Design review of the part shown in the three views and the two pictorial views. Dimensions are in mm from the part's minimum x, y and z. A direction names the side the tool comes from. Round coordinates to 2 decimals unless told otherwise and drop trailing zeros. Loops run counter-clockwise (first coordinate to the right, second up) from the corner with the lowest first, then second, coordinate; pieces in that order, holes last. Notation, with made-up numbers: (-2.75, 55.25) - (11.25, 55.25) arc R20 ccw to (11.25, 84.25) - close; hole circle Ø8 at (82, -31). An arc over 180 degrees is marked (long way). Return JSON: item names as keys, results as strings. Group by question number.
(1) The part is to be moulded in two halves that separate along Z. For the marked faces 3, 4 and 5, say which applies: pulls with the +Z half, pulls with the -Z half, needs draft (parallel to the pull), parting line crosses it, or undercut.
(2) We need section B-B, the plane y = 11. Write out the cut boundary in (x, z), and give its area (3 significant figures).
(3) Clearance check with a flat-ended pin moving along its axis: pin 1 (5 mm diameter, centred on x = 59.5, y = 12, fed in from +Z). State where the tip first meets the part, or that it passes through.
(4) We need section A-A, the plane x = 86. Write out the cut boundary in (y, z).
(5) Wall thickness on L1, parallel to Z at x = 81, y = 4.5; L2, parallel to X at y = 21.25, z = 114.5; L3, parallel to Z at x = 22, y = 20.25: over which ranges is each line inside the solid? List them lowest first. Write a range as [from, to].
(6) We need section D-D, the plane z = 18. Write out the cut boundary in (x, y).
(7) We need section C-C, the plane x = 148. Write out the cut boundary in (y, z).
(8) For the marked faces 1 and 2, list the 3-axis set-ups (+Z, -Z, +X, -X, +Y, -Y) from which the entire face can be reached by the end or side of a thin tool; tool diameter is ignored.
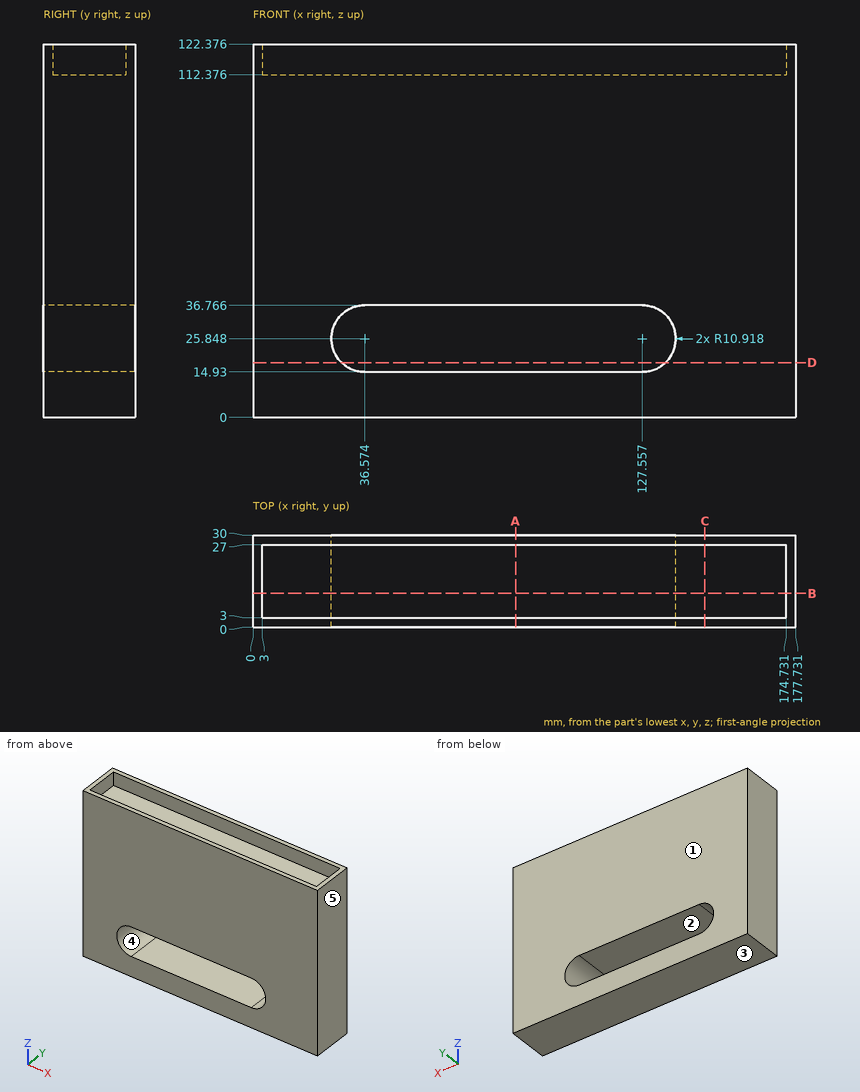
Solutions:
{
 "1": {"face 3": "pulls with the -Z half", "face 4": "undercut", "face 5": "needs draft"},
 "2": {"outline": "(0, 0) - (177.73, 0) - (177.73, 122.38) - (174.73, 122.38) - (174.73, 112.38) - (3, 112.38) - (3, 122.38) - (0, 122.38) - close; hole (36.57, 14.93) - (127.56, 14.93) arc R10.92 ccw to (127.56, 36.77) - (36.57, 36.77) arc R10.92 ccw to start", "area": "17,700 mm^2"},
 "3": {"pin 1": "z = 112.38"},
 "4": {"outline": "(0, 0) - (30, 0) - (30, 14.93) - (0, 14.93) - close; (0, 36.77) - (30, 36.77) - (30, 122.38) - (27, 122.38) - (27, 112.38) - (3, 112.38) - (3, 122.38) - (0, 122.38) - close"},
 "5": {"L1": "[0, 14.93], [36.77, 112.38]", "L2": "[0, 3], [174.73, 177.73]", "L3": "[0, 112.38]"},
 "6": {"outline": "(0, 0) - (28.98, 0) - (28.98, 30) - (0, 30) - close; (135.15, 0) - (177.73, 0) - (177.73, 30) - (135.15, 30) - close"},
 "7": {"outline": "(0, 0) - (30, 0) - (30, 122.38) - (27, 122.38) - (27, 112.38) - (3, 112.38) - (3, 122.38) - (0, 122.38) - close"},
 "8": {"face 1": "+Z, -Z, +X, -X, +Y", "face 2": "+Y, -Y"}
}
